from build123d import *

# Parameters (mm, degrees)
SKETCH1_R           = 4
EXTRUDE1_DEPTH      = 17.5
CHAMFER1_SIZE       = 0.6
SKETCH3_W           = 2
SKETCH3_H           = 1.2
EXTRUDE2_DEPTH      = 18.5
EXTRUDE2_DEPTH_BACK = 18.5


with BuildPart() as part:
    # Sketch1 → Extrude1 (new body, symmetric)
    with BuildSketch(Plane.XY):
        Circle(SKETCH1_R)
    extrude(amount=EXTRUDE1_DEPTH, both=True)

    # Chamfer1
    chamfer1_edges = [part.edges().sort_by_distance(p)[0] for p in [
        (-4, 0, -17.5),
        (-4, 0, 17.5),
    ]]
    chamfer(chamfer1_edges, length=CHAMFER1_SIZE)

    # Sketch3 → Extrude2 (cut, two sides)
    with BuildSketch(Plane.XY) as extrude2_sk:
        with Locations((0, 3.4)):
            Rectangle(SKETCH3_W, SKETCH3_H)
    extrude(amount=EXTRUDE2_DEPTH, mode=Mode.SUBTRACT)
    extrude(extrude2_sk.sketch, amount=-EXTRUDE2_DEPTH_BACK, mode=Mode.SUBTRACT)


solid = part.part
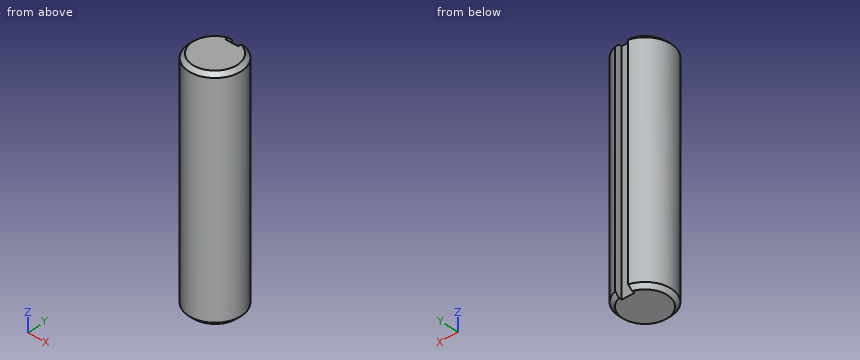
Build history of the part. All positions in model axes, mm. Coordinates: 2 decimals unless noted, no trailing zeros. Write each loop counter-clockwise with the first axis right and the second up, starting at its lowest first coordinate (ties: lowest second). Pieces come first, ordered by that corner, then holes.
(1) Pin check, flat tips, straight feed: pin 1 Ø2 at (y, z) = (-1.5, -11.5) entering from +X; pin 2 Ø0.9 at (y, z) = (3.5, 8) entering from -X; pin 3 Ø2 at (x, z) = (-2.5, -3.5) entering from +Y. Stop position of each tip, or through.
(2) Cut at A-A on x = 0. List the corners of the cut face in (y, z), and give its area (3 significant figures).
(3) Cut at B-B on z = 6. List the corners of the cut face in (x, y), and give its area (3 significant figures).
(4) Drill centre lines: line 1 (Y direction, x = -0.25, z = 4); line 2 (X direction, y = -1.5, z = -6); line 3 (X direction, y = -1, z = -5.5). Where is each one in solid material? Low to high.
Working result:
1. pin 1: stops at x = 3.97
1. pin 2: stops at x = -2.59
1. pin 3: stops at y = 3.71
2. outline: (-4, -16.9) - (-3.4, -17.5) - (2.8, -17.5) - (2.8, 17.5) - (-3.4, 17.5) - (-4, 16.9) - close
2. area: 238 mm2
3. outline: (-1, 2.8) - (-1, 3.87) arc R4 ccw (long way) to (1, 3.87) - (1, 2.8) - close
3. area: 47.9 mm2
4. line 1: y = -3.99 to 2.8
4. line 2: x = -3.71 to 3.71
4. line 3: x = -3.87 to 3.87
